```python
from build123d import *

# Parameters (mm, degrees)
SKETCH1_R               = 21
BOSS_EXTRUDE1_DEPTH     = 8
CUT_EXTRUDE1_DEPTH      = 31.757112998
CUT_EXTRUDE1_DEPTH_BACK = 31.757112998
SKETCH2_R               = 1.3
SKETCH4_R               = 1.1
CUT_EXTRUDE2_DEPTH      = 10
SKETCH5_R               = 1.1
CUT_EXTRUDE3_DEPTH      = 10
SKETCH11_W              = 64
SKETCH11_H              = 66
BOSS_EXTRUDE3_DEPTH     = 10
CUT_EXTRUDE8_START      = -10
SKETCH17_R              = 1.3
CUT_EXTRUDE8_DEPTH      = 10
SKETCH12_W              = 15
SKETCH12_H              = 9
BOSS_EXTRUDE4_DEPTH     = 22
SKETCH13_R              = 1.5
CUT_EXTRUDE4_DEPTH      = 21
SKETCH14_W              = 6
SKETCH14_H              = 41
BOSS_EXTRUDE5_DEPTH     = 22
SKETCH15_R              = 3.2
CUT_EXTRUDE6_DEPTH      = 22
FILLET12_R              = 1
FILLET13_R              = 1
FILLET14_R              = 2.5
SKETCH16_W              = 14
SKETCH16_H              = 5
CUT_EXTRUDE7_DEPTH      = 22
FILLET15_R              = 2.5
SKETCH18_R              = 2.75
CUT_EXTRUDE9_DEPTH      = 3.1


# Some blends are built 0.0001 mm under size
with BuildPart() as part:
    # Sketch1 → Boss-Extrude1 (new body)
    with BuildSketch(Plane.XY):
        Circle(SKETCH1_R)
    extrude(amount=BOSS_EXTRUDE1_DEPTH)

    # Sketch2 → Cut-Extrude1 (cut, two sides: drawn at the far end of the back side and taken through both)
    with BuildSketch(Plane(origin=(0, 0, 0), x_dir=(-1, 0, 0), z_dir=(0, 0, -1)).offset(-CUT_EXTRUDE1_DEPTH_BACK)):
        Circle(SKETCH2_R)
    extrude(amount=CUT_EXTRUDE1_DEPTH + CUT_EXTRUDE1_DEPTH_BACK, mode=Mode.SUBTRACT)

    # Sketch4 → Cut-Extrude2 (cut)
    with BuildSketch(Plane(origin=(0, 0, 0), x_dir=(-1, 0, 0), z_dir=(0, 0, -1))):
        with Locations((16, 0)):
            Circle(SKETCH4_R)
    extrude(amount=-CUT_EXTRUDE2_DEPTH, mode=Mode.SUBTRACT)

    # Sketch5 → Cut-Extrude3 (cut)
    with BuildSketch(Plane(origin=(0, 0, 0), x_dir=(-1, 0, 0), z_dir=(0, 0, -1))):
        with Locations((-16, 0)):
            Circle(SKETCH5_R)
    extrude(amount=-CUT_EXTRUDE3_DEPTH, mode=Mode.SUBTRACT)

    # Sketch11 → Boss-Extrude3 (add)
    with BuildSketch(Plane(origin=(0, 0, 0), x_dir=(-1, 0, 0), z_dir=(0, 0, -1))):
        Rectangle(SKETCH11_W, SKETCH11_H)
    extrude(amount=BOSS_EXTRUDE3_DEPTH)

    # Sketch17 → Cut-Extrude8 (cut)
    with BuildSketch(Plane.XY.offset(CUT_EXTRUDE8_START)):
        with Locations(Location((0, 0, 0), (0, 0, 180))):
            Circle(SKETCH17_R)
    extrude(amount=CUT_EXTRUDE8_DEPTH, mode=Mode.SUBTRACT)

    # Sketch12 → Boss-Extrude4 (add)
    with BuildSketch(Plane(origin=(0, 0, -10), x_dir=(-1, 0, 0), z_dir=(0, 0, -1))):
        with Locations((10.5, -25)):
            Rectangle(SKETCH12_W, SKETCH12_H)
        with Locations((10.5, 25)):
            Rectangle(SKETCH12_W, SKETCH12_H)
    extrude(amount=BOSS_EXTRUDE4_DEPTH)

    # Sketch13 → Cut-Extrude4 (cut)
    with BuildSketch(Plane.ZY.offset(18)):
        with Locations((-25.2, -25.3)):
            Circle(SKETCH13_R)
        with Locations((-15.4, -25.3)):
            Circle(SKETCH13_R)
        with Locations((-25.2, 25.3)):
            Circle(SKETCH13_R)
        with Locations((-15.4, 25.3)):
            Circle(SKETCH13_R)
    extrude(amount=-CUT_EXTRUDE4_DEPTH, mode=Mode.SUBTRACT)

    # Sketch14 → Boss-Extrude5 (add)
    with BuildSketch(Plane(origin=(0, 0, -10), x_dir=(-1, 0, 0), z_dir=(0, 0, -1))):
        with Locations((-21, 0)):
            Rectangle(SKETCH14_W, SKETCH14_H)
    extrude(amount=BOSS_EXTRUDE5_DEPTH)

    # Sketch15 → Cut-Extrude6 (cut)
    with BuildSketch(Plane.ZY.offset(-18)):
        with Locations(Location((-20, 10.5, 0), (0, 0, 270))):
            Circle(SKETCH15_R)
    extrude(amount=-CUT_EXTRUDE6_DEPTH, mode=Mode.SUBTRACT)

    # Fillet12
    fillet12_edges = [part.edges().sort_by_distance(p)[0] for p in [
        (-21, 0, 0),
        (-32, 0, 0),
        (-32, -33, -5),
        (0, 33, 0),
        (-32, 33, -5),
        (32, 0, 0),
        (32, 33, -5),
        (0, -33, 0),
        (32, -33, -5),
        (-32, 0, -10),
        (0, 33, -10),
        (32, 0, -10),
        (0, -33, -10),
    ]]
    fillet(fillet12_edges, radius=FILLET12_R)

    # Fillet13
    fillet13_edges = [part.edges().sort_by_distance(p)[0] for p in [
        (-3, -25, -32),
        (-10.5, -29.5, -32),
        (-18, -25, -32),
        (-10.5, -20.5, -32),
        (-3, 25, -32),
        (-10.5, 20.5, -32),
        (-18, 25, -32),
        (-10.5, 29.5, -32),
        (18, 0, -32),
        (21, 20.5, -32),
        (24, 0, -32),
        (21, -20.5, -32),
    ]]
    fillet(fillet13_edges, radius=FILLET13_R)

    # Fillet14
    # the kernel refuses this fillet: 2.5 mm, written as the material it takes off along each edge
    with BuildSketch(Plane(origin=(21.5, 18, -32), x_dir=(0, 1, 0), z_dir=(-1, 0, 0))) as fillet14_piece_1:
        with BuildLine():
            CenterArc((1.5, -1), 1, 0, 90)
            Line((2.5, -1), (2.5, 0))
            Line((2.5, 0), (1.5, 0))
        make_face()
    revolve(axis=Axis((21.5, 18, -32), (0, 0, -1)), revolution_arc=90, mode=Mode.SUBTRACT)
    with BuildSketch(Plane(origin=(20.5, 18, -32), x_dir=(-1, 0, 0), z_dir=(0, -1, 0))) as fillet14_piece_2:
        with BuildLine():
            CenterArc((1.5, -1), 1, 0, 90)
            Line((2.5, -1), (2.5, 0))
            Line((2.5, 0), (1.5, 0))
        make_face()
    revolve(axis=Axis((20.5, 18, -32), (0, 0, -1)), revolution_arc=90, mode=Mode.SUBTRACT)
    with BuildSketch(Plane(origin=(21.5, -18, -32), x_dir=(1, 0, 0), z_dir=(0, 1, 0))) as fillet14_piece_3:
        with BuildLine():
            CenterArc((1.5, -1), 1, 0, 90)
            Line((2.5, -1), (2.5, 0))
            Line((2.5, 0), (1.5, 0))
        make_face()
    revolve(axis=Axis((21.5, -18, -32), (0, 0, -1)), revolution_arc=90, mode=Mode.SUBTRACT)
    with BuildSketch(Plane(origin=(20.5, -18, -32), x_dir=(0, -1, 0), z_dir=(1, 0, 0))) as fillet14_piece_4:
        with BuildLine():
            CenterArc((1.5, -1), 1, 0, 90)
            Line((2.5, -1), (2.5, 0))
            Line((2.5, 0), (1.5, 0))
        make_face()
    revolve(axis=Axis((20.5, -18, -32), (0, 0, -1)), revolution_arc=90, mode=Mode.SUBTRACT)
    with BuildSketch(Plane(origin=(18, -20.5, -10), x_dir=(0, 1, 0), z_dir=(0, 0, -1)), Plane(origin=(24, -20.5, -10), x_dir=(-1, 0, 0), z_dir=(0, 0, -1)), Plane(origin=(18, 20.5, -10), x_dir=(1, 0, 0), z_dir=(0, 0, -1))) as fillet14_piece_5:
        with BuildLine():
            CenterArc((FILLET14_R, FILLET14_R), FILLET14_R, 180, 90)
            Line((0, FILLET14_R), (0, 0))
            Line((0, 0), (FILLET14_R, 0))
        make_face()
    extrude(amount=22, mode=Mode.SUBTRACT)
    with BuildSketch(Plane(origin=(24, 20.5, -10), x_dir=(-1, 0, 0), z_dir=(0, 0, -1))) as fillet14_piece_6:
        with BuildLine():
            CenterArc((FILLET14_R, -FILLET14_R), FILLET14_R, 90, 90)
            Line((0, -FILLET14_R), (0, 0))
            Line((0, 0), (FILLET14_R, 0))
        make_face()
    extrude(amount=22, mode=Mode.SUBTRACT)
    # the kernel refuses this fillet: 2.5 mm, written as the material it adds along each edge
    with BuildSketch(Plane(origin=(18, 18, -10), x_dir=(-1, 0, 0), z_dir=(0, -1, 0)), Plane(origin=(24, -18, -10), x_dir=(1, 0, 0), z_dir=(0, 1, 0))) as fillet14_2_piece_1:
        with BuildLine():
            CenterArc((FILLET14_R, FILLET14_R), FILLET14_R, 180, 90)
            Line((0, FILLET14_R), (0, 0))
            Line((0, 0), (FILLET14_R, 0))
        make_face()
    extrude(amount=36)
    with BuildSketch(Plane(origin=(21.5, 20.5, -10), x_dir=(0, 1, 0), z_dir=(-1, 0, 0)), Plane(origin=(20.5, -20.5, -10), x_dir=(0, -1, 0), z_dir=(1, 0, 0))) as fillet14_2_piece_2:
        with BuildLine():
            CenterArc((FILLET14_R, FILLET14_R), FILLET14_R, 180, 90)
            Line((0, FILLET14_R), (0, 0))
            Line((0, 0), (FILLET14_R, 0))
        make_face()
    extrude(amount=1)
    with BuildSketch(Plane(origin=(20.5, -18, -10), x_dir=(-1, 0, 0), z_dir=(0, 1, 0))) as fillet14_2_piece_3:
        with BuildLine():
            CenterArc((2.5 + FILLET14_R, -FILLET14_R), FILLET14_R, 90, 90)
            Line((2.5, -FILLET14_R), (2.5, 0))
            Line((2.5, 0), (2.5 + FILLET14_R, 0))
        make_face()
    revolve(axis=Axis((20.5, -18, -10), (0, 0, 1)), revolution_arc=90)
    with BuildSketch(Plane(origin=(21.5, -18, -10), x_dir=(0, -1, 0), z_dir=(-1, 0, 0))) as fillet14_2_piece_4:
        with BuildLine():
            CenterArc((2.5 + FILLET14_R, -FILLET14_R), FILLET14_R, 90, 90)
            Line((2.5, -FILLET14_R), (2.5, 0))
            Line((2.5, 0), (2.5 + FILLET14_R, 0))
        make_face()
    revolve(axis=Axis((21.5, -18, -10), (0, 0, 1)), revolution_arc=90)
    with BuildSketch(Plane(origin=(21.5, 18, -10), x_dir=(0, 1, 0), z_dir=(-1, 0, 0))) as fillet14_2_piece_5:
        with BuildLine():
            CenterArc((2.5 + FILLET14_R, FILLET14_R), FILLET14_R, 180, 90)
            Line((2.5, FILLET14_R), (2.5, 0))
            Line((2.5, 0), (2.5 + FILLET14_R, 0))
        make_face()
    revolve(axis=Axis((21.5, 18, -10), (0, 0, -1)), revolution_arc=90)
    with BuildSketch(Plane(origin=(20.5, 18, -10), x_dir=(0, 1, 0), z_dir=(1, 0, 0))) as fillet14_2_piece_6:
        with BuildLine():
            CenterArc((2.5 + FILLET14_R, -FILLET14_R), FILLET14_R, 90, 90)
            Line((2.5, -FILLET14_R), (2.5, 0))
            Line((2.5, 0), (2.5 + FILLET14_R, 0))
        make_face()
    revolve(axis=Axis((20.5, 18, -10), (0, 0, 1)), revolution_arc=90)

    # Sketch16 → Cut-Extrude7 (cut)
    with BuildSketch(Plane(origin=(0, 0, -10), x_dir=(-1, 0, 0), z_dir=(0, 0, -1))):
        with Locations((-13.170947401, 26.5)):
            Rectangle(SKETCH16_W, SKETCH16_H)
    extrude(amount=-CUT_EXTRUDE7_DEPTH, mode=Mode.SUBTRACT)

    # Fillet15
    fillet15_edges = [part.edges().sort_by_distance(p)[0] for p in [
        (-3, -25, -10),
        (-10.5, -29.5, -10),
        (-18, -25, -10),
        (-3, 25, -10),
        (-18, 25, -10),
        (-10.5, 29.5, -10),
    ]]
    fillet(fillet15_edges, radius=FILLET15_R - 0.0001)  # a hair under: the kernel refuses the full size

    # Sketch18 → Cut-Extrude9 (cut)
    with BuildSketch(Plane(origin=(0, 0, -10), x_dir=(-1, 0, 0), z_dir=(0, 0, -1))):
        Circle(SKETCH18_R)
    extrude(amount=-CUT_EXTRUDE9_DEPTH, mode=Mode.SUBTRACT)


solid = part.part
```
Work out the finished part from the listing and answer in its coordinate system (mm). A direction names the side the tool comes from. Coordinates: 2 decimals unless noted, no trailing zeros. Loops run counter-clockwise (first coordinate to the right, second up) from the corner with the lowest first, then second, coordinate; pieces in that order, holes last. Notation, with made-up numbers: M -32,29.25 L -17,29.25 A27 cw -17,47.25 Z; hole C 39.5,22.25 d7. An arc over 180 degrees is marked long. Use CSV: the item, a comma, the result in double quotes. Start each with the question number.
(1) Find section D-D, the plane x = -7. State how many separate pieces and enclosed holes the cut face has, then the cut area to 3 significant figures.
(2) Consider line 1 (Y direction, x = -8.5, z = -15.4); line 2 (Z direction, x = -12, y = -25); line 3 (Z direction, x = 17, y = 22). Determine where each line is inside the solid, lowest interval first.
(3) For a pull along Y with two mould halves and no side action, classify faces 6 (the face through (-11, 30, -11)), 7 (the face through (0.596, -2.685, -8.472)), 8 (the face through (-18.752, -24.892, -10.713)), 9 (the face through (19, -20, -22)) as +Y half, -Y half, draft (parallel to the pull), parting line (faces both ways), or undercut.
(4) Find section B-B, the plane z = -25.2. Give the vertices of the cut face in (x, y), then the cut area to 3 significant figures.
(5) Find section A-A, the plane y = -25.3. Give the vertices of the cut face in (x, z), then the cut area to 3 significant figures.
(6) Find section C-C, the plane z = -19. Give the vertices of the cut face in (x, y).
(7) For faces 1 (the face through (-18, 25, -22)), 2 (the face through (13, 24, -5)), 3 (the face through (21, -21, -11)), 4 (the face through (-3, 25, -22)), 5 (the face through (17.1, 0, 3.9)), determine the directions among +Z, -Z, +X, -X, +Y, -Y from which every point of the face is accessible in a straight line to the end or side of a thin tool.
(8) Given pin 1 Ø3 at (x, y) = (-20.5, -26) entering from -Z; pin 2 Ø2 at (y, z) = (-22.5, -24.5) entering from +X; pin 3 Ø2 at (y, z) = (23.5, -15) entering from -X; pin 4 Ø2.5 at (y, z) = (25.3, -15.4) entering from -X, each flat-ended and moving along its own axis, determine where each tip first touches the part or whether it passes through.
Recorded:
1,separate pieces,"1"
1,enclosed holes,"4"
1,area,"1,350 mm^2"
2,line 1,"y = -29.5 to -26.8, -23.8 to -20.5, 20.5 to 23.8, 26.8 to 29.5"
2,line 2,"z = -32 to -26.67, -23.73 to -16.87, -13.93 to 0"
2,line 3,"z = -10 to 0"
3,face 6,"+Y half"
3,face 7,"undercut"
3,face 8,"draft"
3,face 9,"-Y half"
4,outline,"M -18,-29.5 L -3,-29.5 L -3,-26.8 L -18,-26.8 Z; M -18,-23.8 L -3,-23.8 L -3,-20.5 L -18,-20.5 Z; M -18,20.5 L -3,20.5 L -3,23.8 L -18,23.8 Z; M -18,26.8 L -3,26.8 L -3,29.5 L -18,29.5 Z; M 18,-18 A2.5 ccw 20.5,-20.5 L 21.5,-20.5 A2.5 ccw 24,-18 L 24,18 A2.5 ccw 21.5,20.5 L 20.5,20.5 A2.5 ccw 18,18 Z"
4,area,"421 mm^2"
5,outline,"M -32,-9 A1 ccw -31,-10 L -20.5,-10 A2.5 cw -18,-12.5 L -18,-13.9 L -3,-13.9 L -3,-12.5 A2.5 cw -0.5,-10 L 31,-10 A1 ccw 32,-9 L 32,-1 A1 ccw 31,0 L -31,0 A1 ccw -32,-1 Z; M -18,-31 A1 ccw -17,-32 L -4,-32 A1 ccw -3,-31 L -3,-26.7 L -18,-26.7 Z; M -18,-23.7 L -3,-23.7 L -3,-16.9 L -18,-16.9 Z"
5,area,"881 mm^2"
6,outline,"M -18,-29.5 L -3,-29.5 L -3,-20.5 L -18,-20.5 Z; M -18,20.5 L -3,20.5 L -3,29.5 L -18,29.5 Z; M 18,-18 A2.5 ccw 20.5,-20.5 L 21.5,-20.5 A2.5 ccw 24,-18 L 24,7.46 L 18,7.46 Z; M 18,13.54 L 24,13.54 L 24,18 A2.5 ccw 21.5,20.5 L 20.5,20.5 A2.5 ccw 18,18 Z"
7,face 1,"-Z, -X, +Y, -Y"
7,face 2,"+Z, -Z"
7,face 3,"-Z, +X, -Y"
7,face 4,"-Z, +X, +Y, -Y"
7,face 5,"+Z"
8,pin 1,"stops at z = -10.5"
8,pin 2,"stops at x = -3"
8,pin 3,"stops at x = -18"
8,pin 4,"passes through"
